from build123d import *

# Parameters (mm, degrees)
F1_DEPTH = 25.4
F2_DEPTH = 3.175
F3_W     = 16.2421034352
F3_H     = 5.08
F4_DEPTH = 54.8132
F5_R     = 3.175


with BuildPart() as f1:
    # F0 (on Right) → F1 (new body)
    with BuildSketch(Plane.YZ):
        with BuildLine():
            Line((-8.1210517176, 8.4002604126), (-8.1210517176, 5.2353069186))
            Line((-8.1210517176, 5.2353069186), (-6.7078045937, 5.2353069186))
            ThreePointArc((-6.7078045937, 5.2353069186), (0, 8.509), (6.7078045937, 5.2353069186))
            Line((6.7078045937, 5.2353069186), (8.1210517176, 5.2353069186))
            Line((8.1210517176, 5.2353069186), (8.1210517176, 8.4002604126))
            ThreePointArc((8.1210517176, 8.4002604126), (0, 11.684), (-8.1210517176, 8.4002604126))
        make_face()
    extrude(amount=F1_DEPTH)



with BuildPart() as f1b:
    # F0 (on Right) → F1, piece 2 (new body)
    with BuildSketch(Plane.YZ):
        with BuildLine():
            Line((-8.1210517176, -5.2353069186), (-8.1210517176, -8.4002604126))
            ThreePointArc((-8.1210517176, -8.4002604126), (0, -11.684), (8.1210517176, -8.4002604126))
            Line((8.1210517176, -8.4002604126), (8.1210517176, -5.2353069186))
            Line((8.1210517176, -5.2353069186), (6.7078045937, -5.2353069186))
            ThreePointArc((6.7078045937, -5.2353069186), (0, -8.509), (-6.7078045937, -5.2353069186))
            Line((-6.7078045937, -5.2353069186), (-8.1210517176, -5.2353069186))
        make_face()
    extrude(amount=F1_DEPTH)


with BuildPart() as f1_1:
    add(f1.part)

    add(f1b.part)  # F2 merges F1b
    # F0 (on Right) → F2 (join)
    with BuildSketch(Plane.YZ):
        with BuildLine():
            Line((-8.1210517176, 5.2353069186), (-8.1210517176, -5.2353069186))
            Line((-8.1210517176, -5.2353069186), (-6.7078045937, -5.2353069186))
            ThreePointArc((-6.7078045937, -5.2353069186), (0, -8.509), (6.7078045937, -5.2353069186))
            Line((6.7078045937, -5.2353069186), (8.1210517176, -5.2353069186))
            Line((8.1210517176, -5.2353069186), (8.1210517176, 5.2353069186))
            Line((8.1210517176, 5.2353069186), (6.7078045937, 5.2353069186))
            ThreePointArc((6.7078045937, 5.2353069186), (0, 8.509), (-6.7078045937, 5.2353069186))
            Line((-6.7078045937, 5.2353069186), (-8.1210517176, 5.2353069186))
        make_face()
        with BuildLine():
            Line((-8.1210517176, 8.4002604126), (-8.1210517176, 5.2353069186))
            Line((-8.1210517176, 5.2353069186), (-6.7078045937, 5.2353069186))
            ThreePointArc((-6.7078045937, 5.2353069186), (0, 8.509), (6.7078045937, 5.2353069186))
            Line((6.7078045937, 5.2353069186), (8.1210517176, 5.2353069186))
            Line((8.1210517176, 5.2353069186), (8.1210517176, 8.4002604126))
            ThreePointArc((8.1210517176, 8.4002604126), (0, 11.684), (-8.1210517176, 8.4002604126))
        make_face()
        with BuildLine():
            Line((-8.1210517176, -5.2353069186), (-8.1210517176, -8.4002604126))
            ThreePointArc((-8.1210517176, -8.4002604126), (0, -11.684), (8.1210517176, -8.4002604126))
            Line((8.1210517176, -8.4002604126), (8.1210517176, -5.2353069186))
            Line((8.1210517176, -5.2353069186), (6.7078045937, -5.2353069186))
            ThreePointArc((6.7078045937, -5.2353069186), (0, -8.509), (-6.7078045937, -5.2353069186))
            Line((-6.7078045937, -5.2353069186), (-8.1210517176, -5.2353069186))
        make_face()
    extrude(amount=-F2_DEPTH)

    # F3 (on face) → F4 (join)
    with BuildSketch(Plane(origin=(-3.175, 0, 0), x_dir=(0, -1, 0), z_dir=(-1, 0, 0))):
        Rectangle(F3_W, F3_H)
    extrude(amount=F4_DEPTH)

    # F5
    f5_edges = [f1_1.edges().sort_by_distance(p)[0] for p in [
        (-3.175, 0, 2.54),
        (-3.175, 0, -2.54),
    ]]
    fillet(f5_edges, radius=F5_R)


solid = f1_1.part
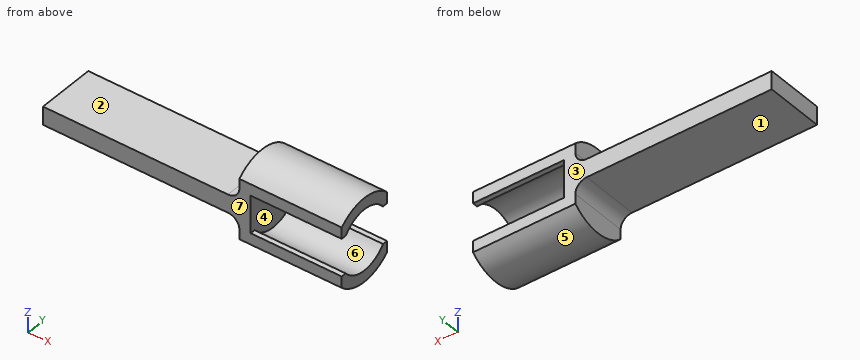
Geometry check sheet. Reference: the model listing, model coordinates, mm. Face numbers are marked on the shaded views. A direction names the side the tool comes from. Give positions to 0.01 mm unless a question says otherwise; leave off trailing zeros. Order: outer loops, then holes, each group sorted by start corner. A loop starts at its lowest first (then second) coordinate and runs counter-clockwise, first axis right, second up.
1) Material ranges on probe 1 along X at (y, z) = (-1.75, -6) (3 decimals); probe 2 along Z at (x, y) = (-10.5, 5.75); probe 3 along X at (y, z) = (1.25, 0.5), recorded low to high.
Results are:
probe 1: x = -3.175 to 0
probe 2: z = -2.54 to 2.54
probe 3: x = -57.99 to 0
2) Cross-section at C-C (z = -6.5). Record the boundary of the cut face in (x, y) (3 decimals).
Results are:
outline: (-3.175, -8.121) - (25.4, -8.121) - (25.4, -5.491) - (0, -5.491) - (0, 5.491) - (25.4, 5.491) - (25.4, 8.121) - (-3.175, 8.121) - close
3) Gauge pin test, flat ends, axial feed: pin 1 (8 mm diameter, centred on x = -29, y = -4, fed in from +Z); pin 2 (1.1 mm diameter, centred on x = 8, y = -7.5, fed in from -Z); pin 3 (3 mm diameter, centred on y = -3.5, z = 7.5, fed in from -X) (3 decimals); pin 4 (8 mm diameter, centred on x = -7.5, z = 7.5, fed in from +Y). Record the tip position at first contact, or that the pin passes through.
Results are:
pin 1: stops at z = 2.54
pin 2: stops at z = -9.39
pin 3: stops at x = -3.175
pin 4: passes through
4) Cross-section at B-B (y = -0.5). Record the boundary of the cut face in (x, z) (3 decimals), then the cut area to 3 significant figures.
Results are:
outline: (-57.988, -2.54) - (-6.35, -2.54) arc R3.175 cw to (-3.175, -5.715) - (-3.175, -11.673) - (25.4, -11.673) - (25.4, -8.494) - (0, -8.494) - (0, 8.494) - (25.4, 8.494) - (25.4, 11.673) - (-3.175, 11.673) - (-3.175, 5.715) arc R3.175 cw to (-6.35, 2.54) - (-57.988, 2.54) - close
area: 518 mm2
5) Cross-section at D-D (x = -52.5). Record the boundary of the cut face in (y, z).
Results are:
outline: (-8.12, -2.54) - (8.12, -2.54) - (8.12, 2.54) - (-8.12, 2.54) - close
6) Tool access check on the marked faces 1, 2, 3 and 4. Record the directions out of +Z, -Z, +X, -X, +Y, -Y that give a thin tool (end or side, any length) a straight path to the whole face; none if there is none.
Results are:
face 1: -Z, -X, +Y, -Y
face 2: +Z, -X, +Y, -Y
face 3: +Z, -Z, +X, -X, +Y
face 4: +X
7) Cross-section at A-A (x = 17). Record the boundary of the cut face in (y, z).
Results are:
outline: (-8.12, -8.4) arc R11.68 ccw to (8.12, -8.4) - (8.12, -5.24) - (6.71, -5.24) arc R8.51 cw to (-6.71, -5.24) - (-8.12, -5.24) - close; (-8.12, 5.24) - (-6.71, 5.24) arc R8.51 cw to (6.71, 5.24) - (8.12, 5.24) - (8.12, 8.4) arc R11.68 ccw to (-8.12, 8.4) - close
8) Draft check along Y on the marked faces 5, 6 and 7. Enter one of: released by +Y, released by -Y, zero draft, split by the parting line, or undercut.
Results are:
face 5: split by the parting line
face 6: undercut
face 7: released by -Y
